Check sheet for the modelled part. Datum: model origin and axes. Units: mm. A direction names the side the tool comes from. Round coordinates to 2 decimals unless told otherwise and drop trailing zeros. Order: outer loops, then holes, each group sorted by start corner. A loop starts at its lowest first (then second) coordinate and runs counter-clockwise, first axis right, second up. Notation, with made-up numbers: (49, 4) -> (81, 4) arc R15 ccw to (81, 32) -> close; hole circle Ø9 at (-25, -12.75). An arc over 180 degrees is marked (long way). Answer in a Markdown table with one row per item. Add a question column.
1. Depth check by flat-ended pin: P1, Ø1.8, axis at x = 0, z = 1.5, coming from the +Y side; P2, Ø1, axis at x = -1.5, y = 3.5, coming from the -Z side; P3, Ø1.5, axis at y = 2, z = 2, coming from the -X side. Enter the tip coordinate at first touch or a pass-through.
2. Sectioned sample at B-B, the plane x = 0. Record the boundary of the cut face in (y, z), then the cut area to 3 significant figures.
3. Access from +Z, -Z, +X, -X, +Y, -Y to the whole of each face (thin tool, end or side, straight path). Record for faces 1 (the cylindrical face through (-0.55, 1.01, -8.01)), 2 (the cylindrical face through (-4.296, 4.028, 0.189)).
4. Sectioned sample at D-D, the plane x = -7. Record the boundary of the cut face in (y, z).
5. Sectioned sample at C-C, the plane z = 8. Record the boundary of the cut face in (x, y).
6. Material ranges on L1, parallel to X at y = 0.8, z = 3.5; L2, parallel to X at y = 0.9, z = 3.75; L3, parallel to Z at x = -0.5, y = 1.9, recorded low to high. Write a range as from..to.
7. Draft check along X on faces 3 (the cylindrical face through (10, 1, 3.2)), 4 (the flat face through (5, 2, 0)), 5 (the flat face through (0, 2, 0)). Enter one of: +X half, -X half, draft (parallel to the pull), parting line (faces both ways), or undercut.
8. Sectioned sample at A-A, the plane z = 0. Record the boundary of the cut face in (x, y).
```python
from build123d import *

# Parameters (mm, degrees)
CUT_EXTRUDE_1_REACH = 4
SKETCH_2_R          = 0.75


with BuildPart() as part:
    # 草图1 → 旋转1 (revolve)
    with BuildSketch(Plane.XY):
        Polygon((0, 0), (10.5, 0), (10.5, 2), (4.3, 2), (4.3, 6), (3, 6), (3, 2), (0, 2), align=None)
    revolve(axis=Axis((0, 2, 0), (0, -1, 0)))

    # 草图2 → 切除-拉伸1 (cut, up to next)
    with BuildSketch(Plane(origin=(0, 2, 0), x_dir=(1, 0, 0), z_dir=(0, 1, 0)), mode=Mode.PRIVATE) as cut_extrude_1_sk1:
        with Locations((3.5, 7.5)):
            Circle(SKETCH_2_R)
    cut_extrude_1_tool1 = extrude(cut_extrude_1_sk1.sketch, amount=-CUT_EXTRUDE_1_REACH, mode=Mode.PRIVATE) & part.part
    add(cut_extrude_1_tool1.solids().sort_by_distance((3.5, 2, -7.5))[0], mode=Mode.SUBTRACT)
    # 草图2 → 切除-拉伸1 (cut, up to next)
    with BuildSketch(Plane(origin=(0, 2, 0), x_dir=(1, 0, 0), z_dir=(0, 1, 0)), mode=Mode.PRIVATE) as cut_extrude_1_sk2:
        with Locations((0, 7.5)):
            Circle(SKETCH_2_R)
    cut_extrude_1_tool2 = extrude(cut_extrude_1_sk2.sketch, amount=-CUT_EXTRUDE_1_REACH, mode=Mode.PRIVATE) & part.part
    add(cut_extrude_1_tool2.solids().sort_by_distance((0, 2, -7.5))[0], mode=Mode.SUBTRACT)
    # 草图2 → 切除-拉伸1 (cut, up to next)
    with BuildSketch(Plane(origin=(0, 2, 0), x_dir=(1, 0, 0), z_dir=(0, 1, 0)), mode=Mode.PRIVATE) as cut_extrude_1_sk3:
        with Locations((-3.5, 7.5)):
            Circle(SKETCH_2_R)
    cut_extrude_1_tool3 = extrude(cut_extrude_1_sk3.sketch, amount=-CUT_EXTRUDE_1_REACH, mode=Mode.PRIVATE) & part.part
    add(cut_extrude_1_tool3.solids().sort_by_distance((-3.5, 2, -7.5))[0], mode=Mode.SUBTRACT)
    # 草图2 → 切除-拉伸1 (cut, up to next)
    with BuildSketch(Plane(origin=(0, 2, 0), x_dir=(1, 0, 0), z_dir=(0, 1, 0)), mode=Mode.PRIVATE) as cut_extrude_1_sk4:
        with Locations((7.5, 3.5)):
            Circle(SKETCH_2_R)
    cut_extrude_1_tool4 = extrude(cut_extrude_1_sk4.sketch, amount=-CUT_EXTRUDE_1_REACH, mode=Mode.PRIVATE) & part.part
    add(cut_extrude_1_tool4.solids().sort_by_distance((7.5, 2, -3.5))[0], mode=Mode.SUBTRACT)
    # 草图2 → 切除-拉伸1 (cut, up to next)
    with BuildSketch(Plane(origin=(0, 2, 0), x_dir=(1, 0, 0), z_dir=(0, 1, 0)), mode=Mode.PRIVATE) as cut_extrude_1_sk5:
        with Locations((7.5, -3.5)):
            Circle(SKETCH_2_R)
    cut_extrude_1_tool5 = extrude(cut_extrude_1_sk5.sketch, amount=-CUT_EXTRUDE_1_REACH, mode=Mode.PRIVATE) & part.part
    add(cut_extrude_1_tool5.solids().sort_by_distance((7.5, 2, 3.5))[0], mode=Mode.SUBTRACT)
    # 草图2 → 切除-拉伸1 (cut, up to next)
    with BuildSketch(Plane(origin=(0, 2, 0), x_dir=(1, 0, 0), z_dir=(0, 1, 0)), mode=Mode.PRIVATE) as cut_extrude_1_sk6:
        with Locations((7.5, 0)):
            Circle(SKETCH_2_R)
    cut_extrude_1_tool6 = extrude(cut_extrude_1_sk6.sketch, amount=-CUT_EXTRUDE_1_REACH, mode=Mode.PRIVATE) & part.part
    add(cut_extrude_1_tool6.solids().sort_by_distance((7.5, 2, 0))[0], mode=Mode.SUBTRACT)
    # 草图2 → 切除-拉伸1 (cut, up to next)
    with BuildSketch(Plane(origin=(0, 2, 0), x_dir=(1, 0, 0), z_dir=(0, 1, 0)), mode=Mode.PRIVATE) as cut_extrude_1_sk7:
        with Locations((3.5, -7.5)):
            Circle(SKETCH_2_R)
    cut_extrude_1_tool7 = extrude(cut_extrude_1_sk7.sketch, amount=-CUT_EXTRUDE_1_REACH, mode=Mode.PRIVATE) & part.part
    add(cut_extrude_1_tool7.solids().sort_by_distance((3.5, 2, 7.5))[0], mode=Mode.SUBTRACT)
    # 草图2 → 切除-拉伸1 (cut, up to next)
    with BuildSketch(Plane(origin=(0, 2, 0), x_dir=(1, 0, 0), z_dir=(0, 1, 0)), mode=Mode.PRIVATE) as cut_extrude_1_sk8:
        with Locations((-3.5, -7.5)):
            Circle(SKETCH_2_R)
    cut_extrude_1_tool8 = extrude(cut_extrude_1_sk8.sketch, amount=-CUT_EXTRUDE_1_REACH, mode=Mode.PRIVATE) & part.part
    add(cut_extrude_1_tool8.solids().sort_by_distance((-3.5, 2, 7.5))[0], mode=Mode.SUBTRACT)
    # 草图2 → 切除-拉伸1 (cut, up to next)
    with BuildSketch(Plane(origin=(0, 2, 0), x_dir=(1, 0, 0), z_dir=(0, 1, 0)), mode=Mode.PRIVATE) as cut_extrude_1_sk9:
        with Locations((0, -7.5)):
            Circle(SKETCH_2_R)
    cut_extrude_1_tool9 = extrude(cut_extrude_1_sk9.sketch, amount=-CUT_EXTRUDE_1_REACH, mode=Mode.PRIVATE) & part.part
    add(cut_extrude_1_tool9.solids().sort_by_distance((0, 2, 7.5))[0], mode=Mode.SUBTRACT)
    # 草图2 → 切除-拉伸1 (cut, up to next)
    with BuildSketch(Plane(origin=(0, 2, 0), x_dir=(1, 0, 0), z_dir=(0, 1, 0)), mode=Mode.PRIVATE) as cut_extrude_1_sk10:
        with Locations((-7.5, -3.5)):
            Circle(SKETCH_2_R)
    cut_extrude_1_tool10 = extrude(cut_extrude_1_sk10.sketch, amount=-CUT_EXTRUDE_1_REACH, mode=Mode.PRIVATE) & part.part
    add(cut_extrude_1_tool10.solids().sort_by_distance((-7.5, 2, 3.5))[0], mode=Mode.SUBTRACT)
    # 草图2 → 切除-拉伸1 (cut, up to next)
    with BuildSketch(Plane(origin=(0, 2, 0), x_dir=(1, 0, 0), z_dir=(0, 1, 0)), mode=Mode.PRIVATE) as cut_extrude_1_sk11:
        with Locations((-7.5, 3.5)):
            Circle(SKETCH_2_R)
    cut_extrude_1_tool11 = extrude(cut_extrude_1_sk11.sketch, amount=-CUT_EXTRUDE_1_REACH, mode=Mode.PRIVATE) & part.part
    add(cut_extrude_1_tool11.solids().sort_by_distance((-7.5, 2, -3.5))[0], mode=Mode.SUBTRACT)
    # 草图2 → 切除-拉伸1 (cut, up to next)
    with BuildSketch(Plane(origin=(0, 2, 0), x_dir=(1, 0, 0), z_dir=(0, 1, 0)), mode=Mode.PRIVATE) as cut_extrude_1_sk12:
        with Locations((-7.5, 0)):
            Circle(SKETCH_2_R)
    cut_extrude_1_tool12 = extrude(cut_extrude_1_sk12.sketch, amount=-CUT_EXTRUDE_1_REACH, mode=Mode.PRIVATE) & part.part
    add(cut_extrude_1_tool12.solids().sort_by_distance((-7.5, 2, 0))[0], mode=Mode.SUBTRACT)


solid = part.part
```
Answer key:
| question | item | result |
|---|---|---|
| 1 | P1 | stops at y = 2 |
| 1 | P2 | stops at z = -4.18 |
| 1 | P3 | stops at x = -10.43 |
| 2 | outline | (0, -10.5) -> (2, -10.5) -> (2, -8.25) -> (0, -8.25) -> close; (0, -6.75) -> (2, -6.75) -> (2, -4.3) -> (6, -4.3) -> (6, -3) -> (2, -3) -> (2, 3) -> (6, 3) -> (6, 4.3) -> (2, 4.3) -> (2, 6.75) -> (0, 6.75) -> close; (0, 8.25) -> (2, 8.25) -> (2, 10.5) -> (0, 10.5) -> close |
| 2 | area | 46.4 mm² |
| 3 | face 1 | +Y, -Y |
| 3 | face 2 | +Y |
| 4 | outline | (0, -7.83) -> (2, -7.83) -> (2, -4.06) -> (0, -4.06) -> close; (0, -2.94) -> (2, -2.94) -> (2, -0.56) -> (0, -0.56) -> close; (0, 0.56) -> (2, 0.56) -> (2, 2.94) -> (0, 2.94) -> close; (0, 4.06) -> (2, 4.06) -> (2, 7.83) -> (0, 7.83) -> close |
| 5 | outline | (-6.8, 0) -> (-4.06, 0) -> (-4.06, 2) -> (-6.8, 2) -> close; (-2.94, 0) -> (-0.56, 0) -> (-0.56, 2) -> (-2.94, 2) -> close; (0.56, 0) -> (2.94, 0) -> (2.94, 2) -> (0.56, 2) -> close; (4.06, 0) -> (6.8, 0) -> (6.8, 2) -> (4.06, 2) -> close |
| 6 | L1 | x = -9.9..-8.25, -6.75..6.75, 8.25..9.9 |
| 6 | L2 | x = -9.81..-8.21, -6.79..6.79, 8.21..9.81 |
| 6 | L3 | z = -10.49..-8.06, -6.94..6.94, 8.06..10.49 |
| 7 | face 3 | parting line |
| 7 | face 4 | draft |
| 7 | face 5 | undercut |
| 8 | outline | (-10.5, 0) -> (-8.25, 0) -> (-8.25, 2) -> (-10.5, 2) -> close; (-6.75, 0) -> (6.75, 0) -> (6.75, 2) -> (4.3, 2) -> (4.3, 6) -> (3, 6) -> (3, 2) -> (-3, 2) -> (-3, 6) -> (-4.3, 6) -> (-4.3, 2) -> (-6.75, 2) -> close; (8.25, 0) -> (10.5, 0) -> (10.5, 2) -> (8.25, 2) -> close |
